Input: part model. Units: mm. Frame: model coordinates. A direction names the side the tool comes from. Round coordinates to 2 decimals unless told otherwise and drop trailing zeros. Order: outer loops, then holes, each group sorted by start corner. A loop starts at its lowest first (then second) coordinate and runs counter-clockwise, first axis right, second up. Notation, with made-up numbers: (46, 46) - (93, 46) arc R22 cw to (93, 85) - close; hole circle Ø1 at (63.5, -19). An arc over 180 degrees is marked (long way). One line per item, written item: value. Start each with the question number.
from build123d import *

# Parameters (mm, degrees)
BOSS_EXTRUDE1_DEPTH = 38
CHAMFER1_SIZE       = 5
CHAMFER2_SIZE       = 1.5


with BuildPart() as part:
    # Sketch1 → Boss-Extrude1 (new body)
    with BuildSketch(Plane(origin=(0, 0, 0), x_dir=(0, 0, -1), z_dir=(1, 0, 0))):
        with BuildLine():
            Line((0, 0), (0, 33))
            ThreePointArc((0, 33), (-0.439339828, 34.060660172), (-1.5, 34.5))
            Line((-1.5, 34.5), (-5.95, 34.5))
            ThreePointArc((-5.95, 34.5), (-7, 35.55), (-5.95, 36.6))
            Line((-5.95, 36.6), (15, 36.6))
            Line((15, 36.6), (15, 35.6))
            Line((15, 35.6), (-5.95, 35.6))
            ThreePointArc((-5.95, 35.6), (-6, 35.55), (-5.95, 35.5))
            Line((-5.95, 35.5), (-1.5, 35.5))
            ThreePointArc((-1.5, 35.5), (0.267766953, 34.767766953), (1, 33))
            Line((1, 33), (1, 0))
            Line((1, 0), (0, 0))
        make_face()
    extrude(amount=BOSS_EXTRUDE1_DEPTH)

    # Chamfer1
    chamfer1_edges = [part.edges().sort_by_distance(p)[0] for p in [
        (0, 36.1, -15),
        (38, 36.1, -15),
    ]]
    chamfer(chamfer1_edges, length=CHAMFER1_SIZE)

    # Chamfer2
    chamfer2_edges = [part.edges().sort_by_distance(p)[0] for p in [
        (0, 0, -0.5),
        (38, 0, -0.5),
    ]]
    chamfer(chamfer2_edges, length=CHAMFER2_SIZE)


solid = part.part
Item 1: Section query C-C on y = 3. Return loops of the section in (x, z), and give its area (3 significant figures).
Item 2: Section query D-D on x = 31. Return loops of the section in (y, z).
Item 3: Section query A-A on z = 4.25. Return loops of the section in (x, y), and give its area (3 significant figures).
Item 4: Line query: L1, parallel to Y at x = 25.5, z = -0.5; L2, parallel to Z at x = 5, y = 32.5; L3, parallel to Y at x = 32.5, z = -7.25. Output: solid intervals per line, ascending.
Item 5: First-contact query: pin 1 Ø1.3 at (x, z) = (13.5, 3.5) entering from -Y; pin 2 Ø1.5 at (x, y) = (30, 11.5) entering from +Z; pin 3 Ø16.5 at (x, y) = (18.5, 22) entering from -Z. Flat tips, straight axial feed; report the tip coordinate or a pass-through.
Item 6: Reachability of faces 5 (the face through (19, 16, 0)), 6 (the face through (2, 36, -12)), 7 (the face through (19, 17, -1)) from +Z, -Z, +X, -X, +Y, -Y: full face, straight path, thin tool, end or side. Return the list, or none.
Item 7: Pull-direction query (Y, two-part tool) for faces 1 (the face through (18.7, 35.5, 7)), 2 (the face through (38, 25.6, -0.3)), 3 (the face through (19, 35, 0)), 4 (the face through (19, 35.6, -5)); classes: released by +Y, released by -Y, zero draft, split by the parting line, or undercut.
Item 8: Section query B-B on x = 2. Return loops of the section in (y, z), and give its area (3 significant figures).
Geometry results:
1. outline: (0, -1) - (38, -1) - (38, 0) - (0, 0) - close
1. area: 38.0 mm^2
2. outline: (0, -1) - (33, -1) arc R2.5 ccw to (35.5, 1.5) - (35.5, 5.95) arc R0.05 cw to (35.6, 5.95) - (35.6, -15) - (36.6, -15) - (36.6, 5.95) arc R1.05 ccw to (34.5, 5.95) - (34.5, 1.5) arc R1.5 cw to (33, 0) - (0, 0) - close
3. outline: (0, 34.5) - (38, 34.5) - (38, 35.5) - (0, 35.5) - close; (0, 35.6) - (38, 35.6) - (38, 36.6) - (0, 36.6) - close
3. area: 76.0 mm^2
4. L1: y = 0 to 34.5, 35.6 to 36.6
4. L2: z = -1 to 0
4. L3: y = 35.6 to 36.6
5. pin 1: stops at y = 34.5
5. pin 2: stops at z = 0
5. pin 3: stops at z = -1
6. face 5: +Z, +X, -X, -Y
6. face 6: -Z, -X, +Y, -Y
6. face 7: -Z, +X, -X, -Y
7. face 1: split by the parting line
7. face 2: zero draft
7. face 3: undercut
7. face 4: undercut
8. outline: (0, -1) - (33, -1) arc R2.5 ccw to (35.5, 1.5) - (35.5, 5.95) arc R0.05 cw to (35.6, 5.95) - (35.6, -12) - (36.6, -12) - (36.6, 5.95) arc R1.05 ccw to (34.5, 5.95) - (34.5, 1.5) arc R1.5 cw to (33, 0) - (0, 0) - close
8. area: 60.3 mm^2
